Verification items for the finished model (mm, model axes). A direction names the side the tool comes from. Give positions to 0.01 mm unless a question says otherwise; leave off trailing zeros. Loops run counter-clockwise (first coordinate to the right, second up) from the corner with the lowest first, then second, coordinate; pieces in that order, holes last. Notation, with made-up numbers: (-40, 66) - (-7, 66) arc R30 cw to (-7, 91) - close; hole circle Ø4 at (77, 79). An arc over 180 degrees is marked (long way). Answer in a Markdown table with one row per item.
```python
from build123d import *

# Parameters (mm, degrees)
F0_W     = 103.5
F0_H     = 9
F1_DEPTH = 2.5
F2_R     = 6.5
F3_W     = 109.5
F3_H     = 12
F4_DEPTH = 1
F5_R     = 8


with BuildPart() as f1:
    # F0 (on Top) → F1 (new body)
    with BuildSketch(Plane.XY):
        with Locations((51.75, -4.5)):
            Rectangle(F0_W, F0_H)
    extrude(amount=F1_DEPTH)

    # F2
    f2_edges = [f1.edges().sort_by_distance(p)[0] for p in [
        (103.5, 0, 1.25),
        (0, 0, 1.25),
    ]]
    fillet(f2_edges, radius=F2_R)

    # F3 (on face) → F4 (join)
    with BuildSketch(Plane(origin=(0, 0, 0), x_dir=(1, 0, 0), z_dir=(0, 0, -1))):
        with Locations((51.75, 3)):
            Rectangle(F3_W, F3_H)
    extrude(amount=F4_DEPTH)

    # F5
    f5_edges = [f1.edges().sort_by_distance(p)[0] for p in [
        (106.5, 3, -0.5),
        (-3, 3, -0.5),
    ]]
    fillet(f5_edges, radius=F5_R)


solid = f1.part
```
Q1. Tool access check on faces 1 (the face through (51, 0, 1)), 2 (the face through (101.646, -1.955, 1.268)), 3 (the face through (0, -8, 1)). Record the directions out of +Z, -Z, +X, -X, +Y, -Y that give a thin tool (end or side, any length) a straight path to the whole face; none if there is none.
Completed:
| item | result |
|---|---|
| face 1 | +Z, +X, -X, +Y |
| face 2 | +Z, +X, +Y |
| face 3 | +Z, -X, +Y, -Y |
Q2. Sectioned sample at C-C (y = -2.5). Record the cut outline in (x, z), and give its area (3 significant figures).
Completed:
| item | result |
|---|---|
| outline | (-2.6, -1) - (106.1, -1) - (106.1, 0) - (102.12, 0) - (102.12, 2.5) - (1.38, 2.5) - (1.38, 0) - (-2.6, 0) - close |
| area | 361 mm^2 |
Q3. Go/stop test with flat-tipped pins: P1, Ø0.8, axis at y = -7.5, z = 1, coming from the +X side; P2, Ø1, axis at x = 63, z = 1, coming from the +Y side; P3, Ø2, axis at y = -1.5, z = -0.5, coming from the +X side. Record where each tip stops, or that it passes through.
Completed:
| item | result |
|---|---|
| P1 | x = 103.5 |
| P2 | y = 0 |
| P3 | x = 106.1 |
Q4. Sectioned sample at B-B (x = 60). Record the cut outline in (y, z).
Completed:
| item | result |
|---|---|
| outline | (-9, -1) - (3, -1) - (3, 0) - (0, 0) - (0, 2.5) - (-9, 2.5) - close |
Q5. Sectioned sample at A-A (z = 1.55). Record the cut outline in (x, y).
Completed:
| item | result |
|---|---|
| outline | (0, -9) - (103.5, -9) - (103.5, -6.5) arc R6.5 ccw to (97, 0) - (6.5, 0) arc R6.5 ccw to (0, -6.5) - close |
Q6. Thickness scan on line 1 (X direction, y = -8, z = 0.05); line 2 (Y direction, x = 31, z = 0.1); line 3 (Z direction, x = 11, y = 0.5). Record the ranges inside material, lowest first.
Completed:
| item | result |
|---|---|
| line 1 | 0 to 103.5 |
| line 2 | -9 to 0 |
| line 3 | -1 to 0 |
